Here's the drawing with two shaded views (mm, measured from the low corner). I have some questions. A direction names the side the tool comes from. Give positions to 0.01 mm unless a question says otherwise; leave off trailing zeros. Order: outer loops, then holes, each group sorted by start corner. A loop starts at its lowest first (then second) coordinate and runs counter-clockwise, first axis right, second up. Notation, with made-up numbers: M 68.25,39.5 L 101.25,39.5 A33 cw 101.25,78.5 Z; hole C 35.25,-13.75 d8. An arc over 180 degrees is marked long. Use a Markdown table: item, result. Add a question column.
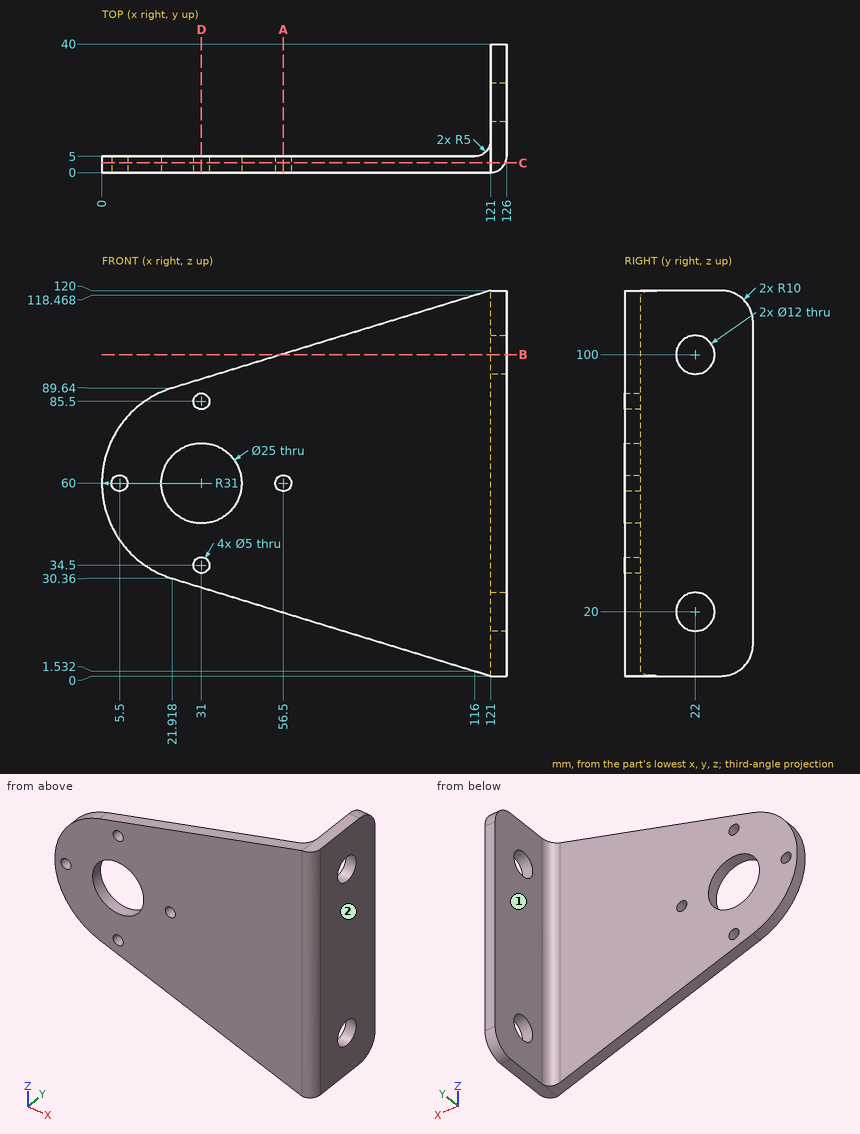
1. If we section it at B-B, the plane z = 100: List the corners of the cut face in (x, y) for me.
2. On a 3-axis mill with a long thin cutter (end or side, diameter ignored), from which of +Z, -Z, +X, -X, +Y, -Y can I reach the whole of each face in a straight line? I mean the marked faces 1 and 2. Say none if no direction works.
3. I need wall thicknesses on L1, parallel to X at y = 2.4, z = 60; L2, parallel to X at y = 3.85, z = 34.5 (1 decimal); L3, parallel to Y at x = 95.5, z = 78. Which ranges of each line are inside material? Lowest first, please. Write a range as [from, to].
4. If we section it at A-A, the plane x = 56.5: List the corners of the cut face in (y, z) for me.
5. If we section it at D-D, the plane x = 31: List the corners of the cut face in (y, z) for me, then the cut area to 3 significant figures.
6. If we section it at C-C, the plane y = 3: List the corners of the cut face in (x, z) for me.
7. Will these pins go through, and if not, where does the flat tip stop? pin 1 (9 mm diameter, centred on y = 26, z = 54, fed in from -X); pin 2 (19 mm diameter, centred on y = 22, z = 100, fed in from +X); pin 3 (6 mm diameter, centred on y = 8.5, z = 52.5, fed in from -X); pin 4 (3 mm diameter, centred on x = 86.5, z = 50, fed in from +Y).
Geometry results:
| question | item | result |
|---|---|---|
| 1 | outline | M 55.73,0 L 121,0 A5 ccw 126,5 L 126,16 L 121,16 L 121,10 A5 cw 116,5 L 55.73,5 Z; M 121,28 L 126,28 L 126,40 L 121,40 Z |
| 2 | face 1 | +Z, -Z, -X, +Y |
| 2 | face 2 | +Z, -Z, +X, +Y, -Y |
| 3 | L1 | x = [0, 3], [8, 18.5], [43.5, 54], [59, 125.27] |
| 3 | L2 | x = [13.4, 28.5], [33.5, 125.9] |
| 3 | L3 | y = [0, 5] |
| 4 | outline | M 0,19.76 L 5,19.76 L 5,57.5 L 0,57.5 Z; M 0,62.5 L 5,62.5 L 5,100.24 L 0,100.24 Z |
| 5 | outline | M 0,27.58 L 5,27.58 L 5,32 L 0,32 Z; M 0,37 L 5,37 L 5,47.5 L 0,47.5 Z; M 0,72.5 L 5,72.5 L 5,83 L 0,83 Z; M 0,88 L 5,88 L 5,92.42 L 0,92.42 Z |
| 5 | area | 149 mm^2 |
| 6 | outline | M 21.92,30.36 L 121,0 L 125.58,0 L 125.58,120 L 121,120 L 21.92,89.64 A31 ccw Z; hole C 5.5,60 d5; hole C 31,60 d25; hole C 31,34.5 d5; hole C 31,85.5 d5; hole C 56.5,60 d5 |
| 7 | pin 1 | stops at x = 121 |
| 7 | pin 2 | stops at x = 126 |
| 7 | pin 3 | stops at x = 118.18 |
| 7 | pin 4 | stops at y = 5 |
